Read the model definition and answer for the solid it produces. Units are mm, in the model's axes. Face numbers are marked on the shaded views. A direction names the side the tool comes from. Give positions to 0.01 mm unless a question says otherwise; leave off trailing zeros. Order: outer loops, then holes, each group sorted by start corner. A loop starts at its lowest first (then second) coordinate and runs counter-clockwise, first axis right, second up. Notation, with made-up numbers: (-35, 21.5) - (9, 21.5) arc R16 cw to (9, 35.5) - close; hole circle Ø6 at (-11, -9.5). An arc over 180 degrees is marked (long way). Write each question's results on one line, items separated by ' | '.
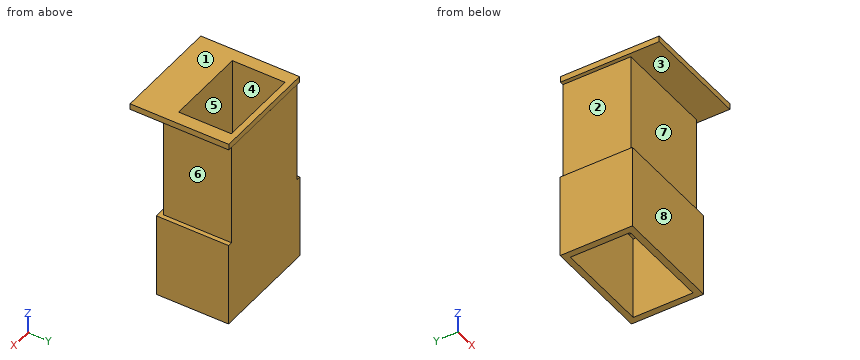
from build123d import *

# Parameters (mm, degrees)
CROQUIS1_W               = 53.24
CROQUIS1_H               = 35.28
CROQUIS1_W_2             = 46.88
CROQUIS1_H_2             = 29.18
SALIENTE_EXTRUIR2_DEPTH  = 41.2
CROQUIS3_W               = 48.88
CROQUIS3_H               = 33.1
CROQUIS3_W_2             = 40.02
CROQUIS3_H_2             = 25.75
SALIENTE_EXTRUIR11_DEPTH = 50
CROQUIS15_W              = 52.73
CROQUIS15_H              = 48.22
CROQUIS15_W_2            = 40.02
CROQUIS15_H_2            = 25.75
SALIENTE_EXTRUIR13_DEPTH = 2.92


with BuildPart() as part:
    # Croquis1 → Saliente-Extruir2 (new body)
    with BuildSketch(Plane.XY):
        with Locations((-10.511813518, 0.307314635)):
            Rectangle(CROQUIS1_W, CROQUIS1_H)
        with Locations((-10.511813518, 0.437314635)):
            Rectangle(CROQUIS1_W_2, CROQUIS1_H_2, mode=Mode.SUBTRACT)
    extrude(amount=SALIENTE_EXTRUIR2_DEPTH)

    # Croquis3 → Saliente-Extruir11 (add)
    with BuildSketch(Plane.XY.offset(41.2)):
        with Locations((-10.511813518, 1.397314635)):
            Rectangle(CROQUIS3_W, CROQUIS3_H)
        with Locations((-10.511813518, 2.152314635)):
            Rectangle(CROQUIS3_W_2, CROQUIS3_H_2, mode=Mode.SUBTRACT)
    extrude(amount=SALIENTE_EXTRUIR11_DEPTH)

    # Croquis15 → Saliente-Extruir13 (add)
    with BuildSketch(Plane.XY.offset(91.2)):
        with Locations((-10.511813518, -6.164685365)):
            Rectangle(CROQUIS15_W, CROQUIS15_H)
        with Locations((-10.511813518, 2.152314635)):
            Rectangle(CROQUIS15_W_2, CROQUIS15_H_2, mode=Mode.SUBTRACT)
    extrude(amount=SALIENTE_EXTRUIR13_DEPTH)


solid = part.part
(1) Each of these flat-tipped pins is pushed along its axis until it touches: pin 1 (14 mm diameter, centred on x = -11.5, z = 29, fed in from -Y); pin 2 (10 mm diameter, centred on y = -15.5, z = 46.5, fed in from -X); pin 3 (7.5 mm diameter, centred on y = 6, z = 58.5, fed in from +X). Where does it stop, or does it pass through?
Conclusion:
pin 1: y = -17.33 | pin 2: x = -34.95 | pin 3: x = 13.93
(2) Section D-D (y = -19.5) is taken. Give the vertices of the cut face in (x, z), plus the area to 3 significant figures.
Conclusion:
outline: (-36.88, 91.2) - (15.85, 91.2) - (15.85, 94.12) - (-36.88, 94.12) - close | area: 154 mm^2
(3) Section C-C (z = 9) is taken. Give the vertices of the cut face in (x, y).
Conclusion:
outline: (-37.13, -17.33) - (16.11, -17.33) - (16.11, 17.95) - (-37.13, 17.95) - close; hole (-33.95, -14.15) - (12.93, -14.15) - (12.93, 15.03) - (-33.95, 15.03) - close
(4) Consider probe 1 along Y at (x, z) = (5, 33.5); probe 2 along X at (y, z) = (13.5, 23.5); probe 3 along Y at (x, z) = (-29, 61). Determine where each line is inside the solid, lowest interval first. Write a range as [from, to].
Conclusion:
probe 1: [-17.33, -14.15], [15.03, 17.95] | probe 2: [-37.13, -33.95], [12.93, 16.11] | probe 3: [-15.15, -10.72], [15.03, 17.95]
(5) Section A-A (y = -6) is taken. Give the vertices of the cut face in (x, z).
Conclusion:
outline: (-37.13, 0) - (-33.95, 0) - (-33.95, 41.2) - (-30.52, 41.2) - (-30.52, 94.12) - (-36.88, 94.12) - (-36.88, 91.2) - (-34.95, 91.2) - (-34.95, 41.2) - (-37.13, 41.2) - close; (9.5, 41.2) - (12.93, 41.2) - (12.93, 0) - (16.11, 0) - (16.11, 41.2) - (13.93, 41.2) - (13.93, 91.2) - (15.85, 91.2) - (15.85, 94.12) - (9.5, 94.12) - close
(6) The mould has two halves that part along Z. Classify the marked faces 1, 2, 3 and 4: pulls with the +Z half, pulls with the -Z half, needs draft (parallel to the pull), parting line crosses it, or undercut.
Conclusion:
face 1: pulls with the +Z half | face 2: undercut | face 3: undercut | face 4: needs draft
(7) For the marked faces 5, 6, 7 and 8, determine the directions among +Z, -Z, +X, -X, +Y, -Y from which every point of the face is accessible in a straight line to the end or side of a thin tool.
Conclusion:
face 5: +Z, -Z | face 6: +X, +Y, -Y | face 7: +X, -X, -Y | face 8: -Z, +X, -X, -Y
